Autodesk Inventor part; units mm, degrees
ref_plane "YZ Plane" through (0, 0, 0) normal (1, 0, 0) x (0, 1, 0)
ref_plane "XZ Plane" through (0, 0, 0) normal (0, 1, 0) x (-1, 0, 0)
ref_plane "XY Plane" through (0, 0, 0) normal (0, 0, 1) x (1, 0, 0)
sketch "Sketch1" plane through (0, 0, 0) normal (0, 0, 1) x (1, 0, 0)
  circle A0 centre (0, 0) radius 5
  dimension "d0" = 10
extrude "Extrusion1" add sketch "Sketch1" along normal blind 15
sketch "Sketch2" plane through (0, 0, 15) normal (0, 0, 1) x (1, 0, 0)
  line L0 (-4.9749, -0.5) -> (4.9749, -0.5)
  line L1 (4.9749, -0.5) -> (4.9749, 0.5)
  line L2 (4.9749, 0.5) -> (-4.9749, 0.5)
  line L3 (-4.9749, 0.5) -> (-4.9749, -0.5)
  circle A0 centre (0, 0) radius 5
  dimension "d3" = 1
sketch "Sketch3" plane through (0, 0, 0) normal (0, 0, -1) x (-1, 0, 0)
  circle A0 centre (0, 0) radius 1.4142
hole "Hole1" at (0, 0, 0) direction (0, 0, 1) diameter 3.302 depth 7
extrude "Extrusion2" add sketch "Sketch2" along normal blind 2 contours L3 L2 L1 L0
ref_plane "Work Plane1" through (-4.9749, 5, 15) normal (0, 1, 0) x (1, 0, 0)
ref_plane "Work Plane2" through (-4.9749, -5, 15) normal (0, -1, 0) x (1, 0, 0)
sketch "Sketch5" plane through (-4.9749, -5, 15) normal (0, -1, 0) x (1, 0, 0)
  circle A0 centre (5, -4) radius 1.0003
  line L0 (9.9499, 0) -> (0, 0)
  point P0 (4.9749, -15)
  dimension "d16" = 4
hole "Hole2" at (0.0251, -5, 11) direction (0, 1, 0) diameter 3.302 depth 4.5
sketch "Sketch6" plane through (0, 0, 15) normal (0, 0, 1) x (1, 0, 0)
  arc A0 (-4.9749, 0.5) -> (-4.9749, -0.5) centre (0, 0) ccw
  line L0 (4.9749, 0.5) -> (4.9749, -0.5)
  line L1 (-4.9749, -0.5) -> (4.9749, -0.5)
  line L2 (4.9749, -0.5) -> (4.9749, 0.5)
  line L3 (4.9749, 0.5) -> (-4.9749, 0.5)
  line L4 (-4.9749, 0.5) -> (-4.9749, -0.5)
extrude "Extrusion3" add sketch "Sketch6" against normal blind 2 contours L3 L0 L1 L4
sketch "Sketch7" plane through (0, 0, 17) normal (0, 0, 1) x (1, 0, 0)
  line L0 (5, 0.6) -> (-5, 0.6)
  line L1 (-5, 0.6) -> (-5, -0.6)
  line L2 (-5, -0.6) -> (5, -0.6)
  line L3 (5, -0.6) -> (5, 0.6)
  arc A0 (4.9749, -0.5) -> (4.9749, 0.5) centre (0, 0) ccw
  arc A1 (-4.9749, 0.5) -> (-4.9749, -0.5) centre (0, 0) ccw
  dimension "d35" = 1.2
  dimension "d36" = 0.6
extrude "Extrusion4" cut sketch "Sketch7" against normal blind 10
properties part number "slit-adapter-clear-scope_8_2018"
Geometry check sheet. Reference: the model listing, model coordinates, mm. A direction names the side the tool comes from. Round coordinates to 2 decimals unless told otherwise and drop trailing zeros. Write each loop counter-clockwise with the first axis right and the second up, starting at its lowest first coordinate (ties: lowest second). Pieces come first, ordered by that corner, then holes.
Item 1: Material ranges on line 1 along X through (y, z) = (0, 5); line 2 along Y through (x, z) = (0.5, 3); line 3 along X through (y, z) = (-4.05, 11), recorded low to high.
Determined:
line 1: x = -5 to -1.65, 1.65 to 5
line 2: y = -4.97 to -1.57, 1.57 to 4.97
line 3: x = -2.93 to -1.63, 1.68 to 2.93
Item 2: Section check D-D (y = 1.25). Record the boundary of the cut face in (x, z).
Determined:
outline: (-4.84, 0) - (-1.08, 0) - (-1.08, 7) - (1.08, 7) - (1.08, 0) - (4.84, 0) - (4.84, 15) - (-4.84, 15) - close
Item 3: Go/stop test with flat-tipped pins: pin 1 Ø5 at (y, z) = (-1.5, 9) entering from +X; pin 2 Ø4 at (y, z) = (-3.5, 6) entering from -X; pin 3 Ø1.5 at (x, z) = (2, 6) entering from -Y. Record where each tip stops, or that it passes through.
Determined:
pin 1: stops at x = 5
pin 2: stops at x = -4.77
pin 3: stops at y = -4.84
Item 4: Mould release check, pull along Z, two halves, no side actions. Record for faces 4 (the face through (0, -2, 15)), 5 (the face through (-1.367, -2.769, 10.112)), 6 (the face through (0, -1, 7)), 7 (the face through (0, -0.6, 13)): +Z half, -Z half, draft (parallel to the pull), parting line (faces both ways), or undercut.
Determined:
face 4: +Z half
face 5: undercut
face 6: -Z half
face 7: draft
Item 5: Access from +Z, -Z, +X, -X, +Y, -Y to the whole of each face (thin tool, end or side, straight path). Record for faces 1 (the face through (-3, 0, 7)), 2 (the face through (0.632, 1.525, 3.549)), 3 (the face through (4.619, 1.915, 7.395)).
Determined:
face 1: +Z, +X, -X
face 2: -Z
face 3: +Z, -Z
Item 6: Section check A-A (y = 0). Record the boundary of the cut face in (x, z).
Determined:
outline: (-5, 0) - (-1.65, 0) - (-1.65, 7) - (-5, 7) - close; (1.65, 0) - (5, 0) - (5, 7) - (1.65, 7) - close
Item 7: Section check C-C (x = -4). Record the boundary of the cut face in (y, z).
Determined:
outline: (-3, 0) - (3, 0) - (3, 15) - (0.6, 15) - (0.6, 7) - (-0.6, 7) - (-0.6, 15) - (-3, 15) - close
Item 8: Section check B-B (z = 11). Record the boundary of the cut face in (x, y), plus the area to 3 significant figures.
Determined:
outline: (-4.96, -0.6) arc R5 ccw to (-1.63, -4.73) - (-1.63, -0.6) - close; (-4.96, 0.6) - (4.96, 0.6) arc R5 ccw to start; (1.68, -4.71) arc R5 ccw to (4.96, -0.6) - (1.68, -0.6) - close
area: 52.3 mm2
